Geometry: see drawing. Coordinates: mm, zero at the bounding-box minimum. A direction names the side the tool comes from. Give positions to 0.01 mm unless a question says otherwise; leave off trailing zeros. Return JSON: item names as keys, results as strings. Group by question number.
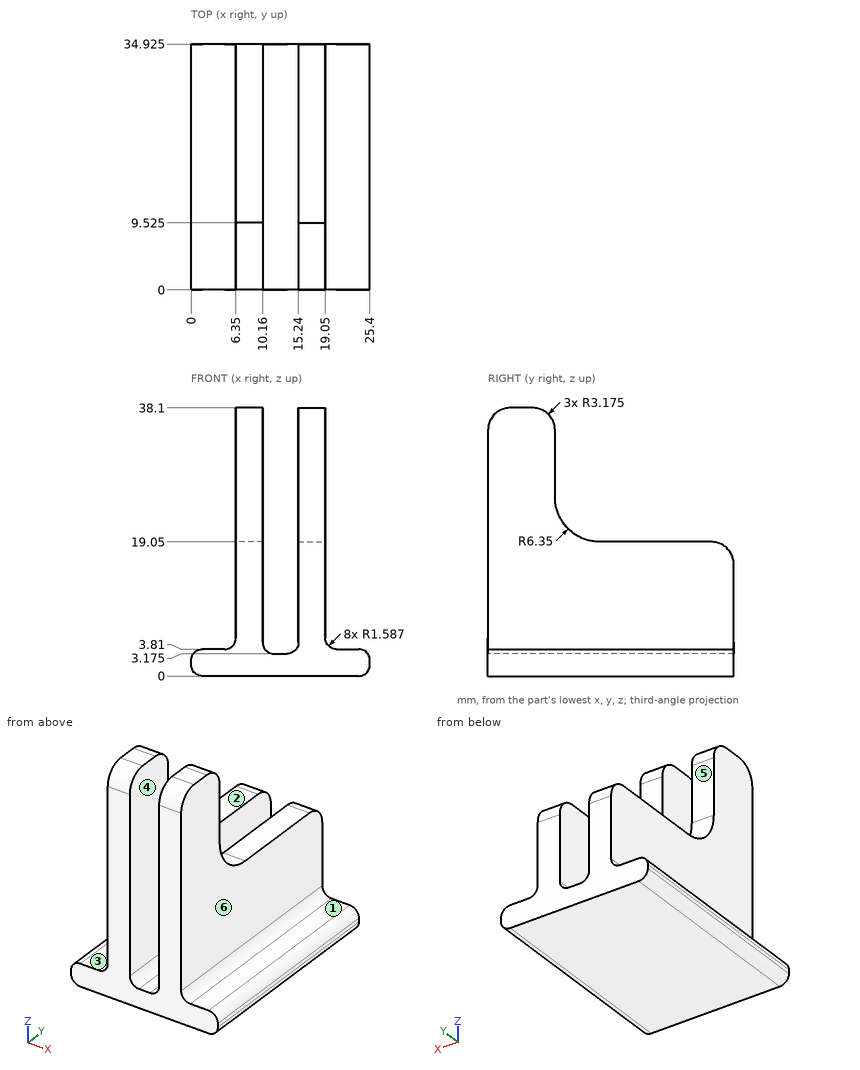
Item 1: Pull-direction query (X, two-part tool) for the marked faces 4, 5 and 6; classes: pulls with the +X half, pulls with the -X half, needs draft (parallel to the pull), parting line crosses it, or undercut.
Item 2: Reachability of the marked faces 1, 2 and 3 from +Z, -Z, +X, -X, +Y, -Y: full face, straight path, thin tool, end or side. Return the list, or none.
Item 3: First-contact query: pin 1 Ø2 at (x, y) = (13, 20) entering from +Z; pin 2 Ø4 at (x, z) = (8.5, 29.5) entering from +Y (1 decimal); pin 3 Ø4 at (x, y) = (4.5, 17.5) entering from +Z. Flat tips, straight axial feed; report the tip coordinate or a pass-through.
Item 4: Material intervals for line 1 (X direction, y = 15, z = 9); line 2 (Z direction, x = 10, y = 29); line 3 (Z direction, x = 20.75, y = 30.5), sorted ascending. Write a range as from..to.
Answer below:
{
 "1": {"face 4": "undercut", "face 5": "needs draft", "face 6": "pulls with the +X half"},
 "2": {"face 1": "+Z, +X, +Y, -Y", "face 2": "+Z, +X, -X, +Y", "face 3": "+Z, -X, +Y, -Y"},
 "3": {"pin 1": "z = 3.21", "pin 2": "y = 9.5", "pin 3": "z = 19.05"},
 "4": {"line 1": "6.35..10.16, 15.24..19.05", "line 2": "0..19.05", "line 3": "0..3.81"}
}
